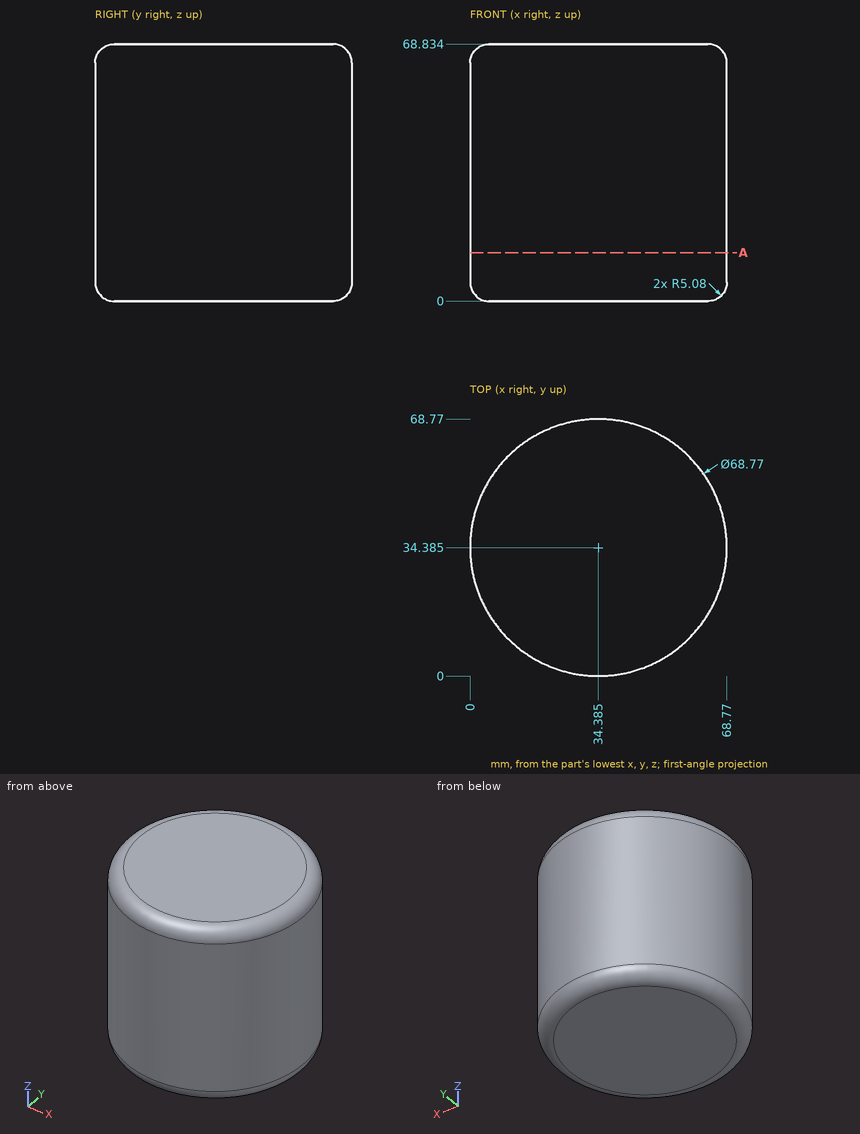
Geometry: see drawing. Coordinates: mm, zero at the bounding-box minimum. Coordinates: 2 decimals unless noted, no trailing zeros. Loops run counter-clockwise (first coordinate to the right, second up) from the corner with the lowest first, then second, coordinate; pieces in that order, holes last.
(1) Material intervals for probe 1 along X at (y, z) = (34, 45.5); probe 2 along X at (y, z) = (60.5, 16); probe 3 along Y at (x, z) = (9, 33), sorted ascending.
(2) First-contact query: pin 1 Ø1.5 at (x, y) = (58.5, 10) entering from -Z; pin 2 Ø2 at (y, z) = (58, 19) entering from -X; pin 3 Ø6 at (y, z) = (25, 56) entering from +X. Flat tips, straight axial feed; report the tip coordinate or a pass-through.
(3) Section A-A on z = 13. Return the cut outline in (x, y) (1 decimal).
Data:
1. probe 1: x = 0 to 68.77
1. probe 2: x = 12.02 to 56.75
1. probe 3: y = 11.19 to 57.58
2. pin 1: stops at z = 2.28
2. pin 2: stops at x = 8.48
2. pin 3: stops at x = 68.17
3. outline: circle Ø68.8 at (34.4, 34.4)
